The figure shows three views and two pictorial views of one solid part (mm, origin at its lowest corner). Answer the questions. Round coordinates to 2 decimals unless told otherwise and drop trailing zeros. Order: outer loops, then holes, each group sorted by start corner. A loop starts at its lowest first (then second) coordinate and runs counter-clockwise, first axis right, second up. Notation, with made-up numbers: (14.5, -22.75) - (71.5, -22.75) arc R22 cw to (71.5, 14.25) - close; hole circle Ø1 at (-2, 13.25). An arc over 180 degrees is marked (long way). Use CSV: the item, a comma, the result in double quotes.
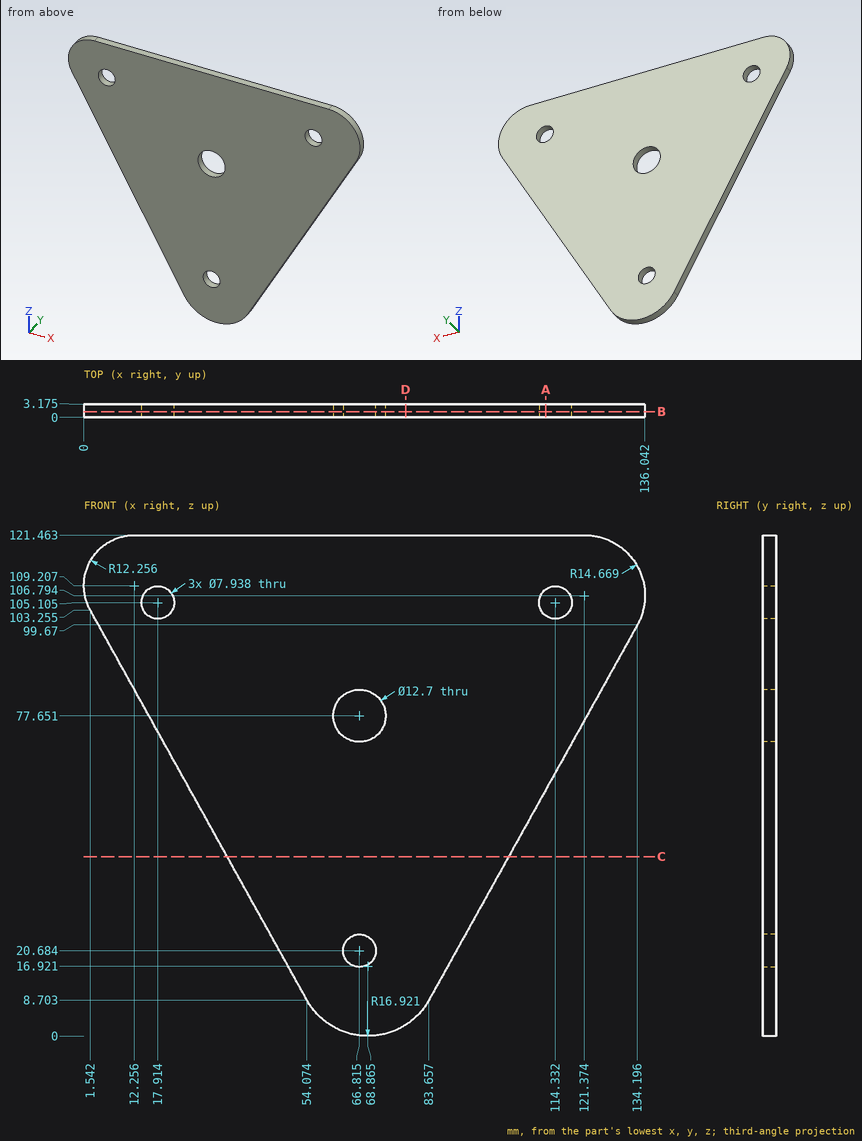
(1) Find section A-A (x = 112). Determine the outline of the cut face in (y, z) (1 decimal).
Findings below:
outline,"(0, 59.7) - (3.2, 59.7) - (3.2, 101.9) - (0, 101.9) - close; (0, 108.3) - (3.2, 108.3) - (3.2, 121.5) - (0, 121.5) - close"
(2) Find the intervals of material crossed by L1, parallel to X at y = 2.85, z = 19 (1 decimal); L2, parallel to X at y = 0.1, z = 73.5 (1 decimal); L3, parallel to Z at x = 74, y = 0.85, in increasing order. Write a range as from..to.
Findings below:
L1,"x = 48.4..63.2, 70.4..89.4"
L2,"x = 18.1..62, 71.6..119.7"
L3,"z = 0.8..121.46"
(3) Each of these flat-tipped pins is pushed along its axis until it touches: pin 1 (1.5 mm diameter, centred on y = 2.5, z = 104, fed in from +X); pin 2 (14.5 mm diameter, centred on x = 66.81, z = 77.65, fed in from +Y) (1 decimal); pin 3 (1 mm diameter, centred on x = 73.5, y = 1.5, fed in from -Z); pin 4 (1.5 mm diameter, centred on y = 0.5, z = 49.5, fed in from +X). Where does it stop, or does it pass through?
Findings below:
pin 1,"stops at x = 135.9"
pin 2,"stops at y = 3.2"
pin 3,"stops at z = 0.51"
pin 4,"stops at x = 106.74"
(4) Find section D-D (x = 78). Determine the outline of the cut face in (y, z) (1 decimal), and give its area (3 significant figures).
Findings below:
outline,"(0, 2.7) - (3.2, 2.7) - (3.2, 121.5) - (0, 121.5) - close"
area,"377 mm²"
(5) Find section B-B (y = 1.3). State how many separate pieces and enclosed holes the cut face has, and give its area (3 significant figures).
Findings below:
separate pieces,"1"
enclosed holes,"4"
area,"10,100 mm²"
(6) Find section C-C (z = 43.5). Determine the outline of the cut face in (x, y) (1 decimal), and give its area (3 significant figures).
Findings below:
outline,"(34.7, 0) - (103, 0) - (103, 3.2) - (34.7, 3.2) - close"
area,"217 mm²"
